```python
from build123d import *

# Parameters (mm, degrees)
F0_R     = 100
F1_DEPTH = 120
F2_R     = 20


with BuildPart() as f1:
    # F0 (on Front) → F1 (new body)
    with BuildSketch(Plane.XZ):
        Circle(F0_R)
    extrude(amount=F1_DEPTH)

    # F2
    f2_edges = [f1.edges().sort_by_distance(p)[0] for p in [
        (-100, -120, 0),
    ]]
    fillet(f2_edges, radius=F2_R)

    # F3: F1 across face


with BuildPart() as f1_1:
    add(f1.part)
    add(f1.part.mirror(Plane(origin=(0, 0, 0), x_dir=(1, 0, 0), z_dir=(0, 1, 0))))


solid = f1_1.part
```
Geometry check sheet. Reference: the model listing, model coordinates, mm. Give positions to 0.01 mm unless a question says otherwise; leave off trailing zeros. Write each loop counter-clockwise with the first axis right and the second up, starting at its lowest first coordinate (ties: lowest second). Pieces come first, ordered by that corner, then holes. Notation, with made-up numbers: (88.5, 2) - (98.5, 2) arc R27 ccw to (98.5, 27) - close; hole circle Ø11 at (52.25, 8.5). An arc over 180 degrees is marked (long way). Use a Markdown table: item, result.
Q1. Thickness scan on L1, parallel to Z at x = -1, y = -74 (3 decimals); L2, parallel to Z at x = -6.5, y = 2.5; L3, parallel to X at y = -79, z = 86. Record the ranges inside material, lowest first. Write a range as [from, to].
Computed:
| item | result |
|---|---|
| L1 | z = [-99.995, 99.995] |
| L2 | z = [-99.79, 99.79] |
| L3 | x = [-51.03, 51.03] |
Q2. Go/stop test with flat-tipped pins: P1, Ø6, axis at y = 81, z = 16.5, coming from the -X side; P2, Ø10, axis at y = 13, z = 43.5, coming from the +X side; P3, Ø8, axis at x = -60, z = -65, coming from the -Y side. Record where each tip stops, or that it passes through.
Computed:
| item | result |
|---|---|
| P1 | stops at x = -99.08 |
| P2 | stops at x = 92.29 |
| P3 | stops at y = -119.5 |
Q3. Section check A-A, the plane y = 17. Enter the section's corners in (x, z).
Computed:
| item | result |
|---|---|
| outline | circle Ø200 at (0, 0) |
